```python
from build123d import *

# Parameters (mm, degrees)
FILLET1_R = 0.2
FILLET2_R = 0.2


with BuildPart() as part:
    # Sketch1 → Revolve1 (revolve)
    with BuildSketch(Plane.XY):
        with BuildLine():
            Line((0, 0), (-6.05, 0))
            Line((-6.05, 0), (-6.05, 3.803589838))
            Line((-6.05, 3.803589838), (-5.85, 4.15))
            Line((-5.85, 4.15), (-5.85, 5.2))
            ThreePointArc((-5.85, 5.2), (-5.791421356, 5.341421356), (-5.65, 5.4))
            Line((-5.65, 5.4), (0, 5.4))
            Line((0, 5.4), (0, 0))
        make_face()
    revolve(axis=Axis((0, 5.4, 0), (0, -1, 0)))

    # Fillet1
    fillet1_edges = [part.edges().sort_by_distance(p)[0] for p in [
        (6.05, 0, 0),
    ]]
    fillet(fillet1_edges, radius=FILLET1_R)

    # Fillet2
    fillet2_edges = [part.edges().sort_by_distance(p)[0] for p in [
        (5.85, 4.15, 0),
        (6.05, 3.803589838, 0),
    ]]
    fillet(fillet2_edges, radius=FILLET2_R)


solid = part.part
```
The model under review builds one solid part; all positions refer to its coordinate system, in mm. A direction names the side the tool comes from. Round coordinates to 2 decimals unless told otherwise and drop trailing zeros. Write each loop counter-clockwise with the first axis right and the second up, starting at its lowest first coordinate (ties: lowest second). Pieces come first, ordered by that corner, then holes.
(1) We need section A-A on y = 0.9. Give the boundary of the cut face in (x, z).
(2) We need section B-B on y = 4.8. Give the boundary of the cut face in (x, z), and give its area (3 significant figures).
(3) Machinability: for faces 1 (the flat face through (0, 0, 0)), 2 (the cylindrical face through (1.27, 4.71, 5.71)), which of the approach directions +Z, -Z, +X, -X, +Y, -Y give a long, thin tool a straight path to every point of the face, cutting with its end or side? Answer none if there is none.
(4) Insertion check: pin 1 (1.5 mm diameter, centred on y = 3.5, z = 4, fed in from -X); pin 2 (2 mm diameter, centred on x = -2.5, y = 2, fed in from -Z). Each pin has a flat end and moves straight along its axis. Give the tip position at first contact, or say it passes through.
(5) Wall thickness on L1, parallel to Y at x = -5.5, z = 1.5; L2, parallel to X at y = 1, z = -1; L3, parallel to Z at x = -2, y = 0.6: over which ranges is each line inside the solid? List them lowest first.
Findings below:
1. outline: circle Ø12.1 at (0, 0)
2. outline: circle Ø11.7 at (0, 0)
2. area: 108 mm2
3. face 1: +Z, -Z, +X, -X, -Y
3. face 2: +Y
4. pin 1: stops at x = -5.1
4. pin 2: stops at z = -5.86
5. L1: y = 0 to 5.39
5. L2: x = -5.97 to 5.97
5. L3: z = -5.71 to 5.71
